Design review of the part built by this model. Coordinates are the model's own, in mm. Round coordinates to 2 decimals unless told otherwise and drop trailing zeros. Write each loop counter-clockwise with the first axis right and the second up, starting at its lowest first coordinate (ties: lowest second). Pieces come first, ordered by that corner, then holes. Notation, with made-up numbers: (-17.75, 62) -> (1.25, 62) arc R25 cw to (1.25, 85) -> close; hole circle Ø7 at (0.25, -14.5). An arc over 180 degrees is marked (long way). One line per question, with ' | ' between items. Start each with the question number.
1) For probe 1 along Y at (x, z) = (50.8, 0) (3 decimals); probe 2 along Y at (x, z) = (-44.5, 2.5) (3 decimals); probe 3 along X at (y, z) = (84.5, 2.5), list the stretches that pass through material, from the lowest coordinate up.
2) Consider section A-A (z = 0). Give the boundary of the cut face in (x, y) (3 decimals), then the cut area to 3 significant figures.
3) Consider section C-C (y = 78.5). Give the boundary of the cut face in (x, z) (3 decimals), then the cut area to 3 significant figures.
4) Consider section B-B (x = -118.5). Give the boundary of the cut face in (y, z) (3 decimals).
5) Insertion check: pin 1 Ø1 at (x, z) = (-61, 2) entering from -Y; pin 2 Ø17.5 at (x, y) = (50.8, 34.925) entering from +Z; pin 3 Ø1.5 at (y, z) = (-93, -2) entering from -X. Each pin has a flat end and moves straight along its axis. Give the tip position at first contact, or say it passes through.
```python
from build123d import *

# Parameters (mm, degrees)
SKETCH1_R           = 10.795
BOSS_EXTRUDE1_DEPTH = 3.175
FILLET1_R           = 25.4
FILLET2_R           = 78.74


with BuildPart() as part:
    # Sketch1 → Boss-Extrude1 (new, symmetric)
    with BuildSketch(Plane.XY):
        Polygon((-63.5, 155.575), (-185.951039645, 9.643533586), (-63.5, -155.575), (63.5, -155.575), (185.951039645, 9.643533586), (63.5, 155.575), align=None)
        with Locations((-50.8, 34.925)):
            Circle(SKETCH1_R, mode=Mode.SUBTRACT)
        with Locations((50.8, 34.925)):
            Circle(SKETCH1_R, mode=Mode.SUBTRACT)
    extrude(amount=BOSS_EXTRUDE1_DEPTH, both=True)

    # Fillet1
    fillet1_edges = [part.edges().sort_by_distance(p)[0] for p in [
        (63.5, 155.575, 0),
        (63.5, -155.575, 0),
        (-63.5, -155.575, 0),
        (-63.5, 155.575, 0),
    ]]
    fillet(fillet1_edges, radius=FILLET1_R)

    # Fillet2
    fillet2_edges = [part.edges().sort_by_distance(p)[0] for p in [
        (185.951039645, 9.643533586, 0),
        (-185.951039645, 9.643533586, 0),
    ]]
    fillet(fillet2_edges, radius=FILLET2_R)


solid = part.part
```
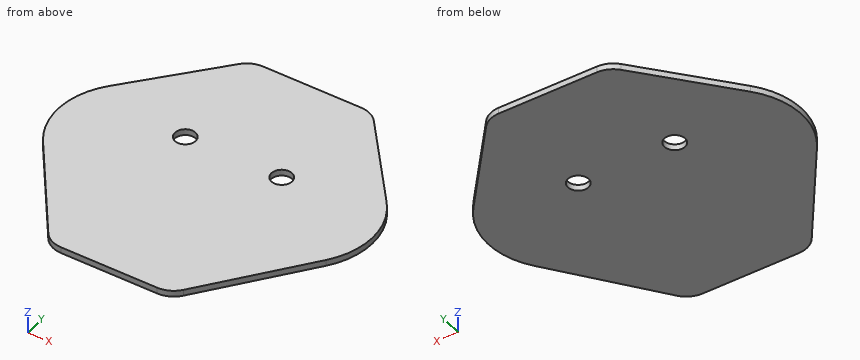
From the geometry:
1) probe 1: y = -155.575 to 24.13, 45.72 to 155.575 | probe 2: y = -155.575 to 26.159, 43.691 to 155.575 | probe 3: x = -123.14 to 123.14
2) outline: (-148.961, -40.266) -> (-71.116, -145.299) arc R25.4 ccw to (-50.71, -155.575) -> (50.71, -155.575) arc R25.4 ccw to (71.116, -145.299) -> (148.961, -40.266) arc R78.74 ccw to (146.019, 57.232) -> (71.113, 146.502) arc R25.4 ccw to (51.656, 155.575) -> (-51.656, 155.575) arc R25.4 ccw to (-71.113, 146.502) -> (-146.019, 57.232) arc R78.74 ccw to start; hole circle Ø21.59 at (-50.8, 34.925); hole circle Ø21.59 at (50.8, 34.925) | area: 75,300 mm2
3) outline: (-128.174, -3.175) -> (128.174, -3.175) -> (128.174, 3.175) -> (-128.174, 3.175) -> close | area: 1,630 mm2
4) outline: (-81.366, -3.175) -> (90.029, -3.175) -> (90.029, 3.175) -> (-81.366, 3.175) -> close
5) pin 1: stops at y = -153.61 | pin 2: passes through | pin 3: stops at x = -110.43
